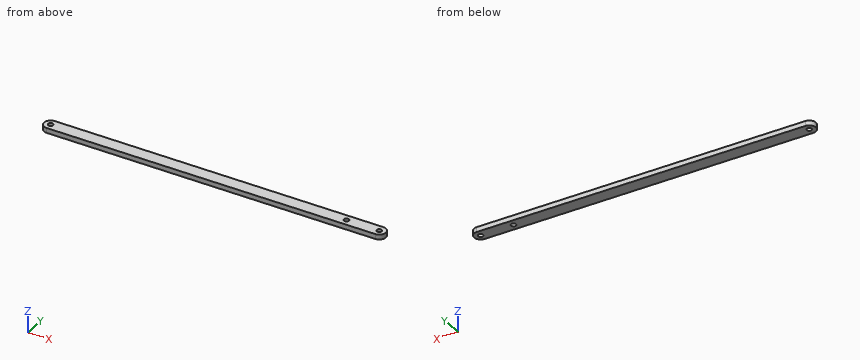
```python
from build123d import *

# Parameters (mm, degrees)
SKETCH1_R           = 3
BOSS_EXTRUDE1_DEPTH = 6
SCALE1_SCALE        = 0.5


with BuildPart() as part:
    # Sketch1 → Boss-Extrude1 (new body)
    with BuildSketch(Plane.XY):
        with BuildLine():
            Line((-200, 8), (200, 8))
            ThreePointArc((200, 8), (208, 0), (200, -8))
            Line((200, -8), (-200, -8))
            ThreePointArc((-200, -8), (-208, 0), (-200, 8))
        make_face()
        with Locations((-200, 0)):
            Circle(SKETCH1_R, mode=Mode.SUBTRACT)
        with Locations((200, 0)):
            Circle(SKETCH1_R, mode=Mode.SUBTRACT)
        with Locations((160, 0)):
            Circle(SKETCH1_R, mode=Mode.SUBTRACT)
    extrude(amount=-BOSS_EXTRUDE1_DEPTH)


with BuildPart() as part_1:
    # Scale1: scaled about (-0.694249163, 0, -3)
    add(part.part.scale(SCALE1_SCALE).moved(Location((-0.347124581, 0, -1.5))))


solid = part_1.part
```
CAD build for the part. Positions are in the model's coordinates, mm. Give positions to 0.01 mm unless a question says otherwise; leave off trailing zeros. Write each loop counter-clockwise with the first axis right and the second up, starting at its lowest first coordinate (ties: lowest second). Pieces come first, ordered by that corner, then holes. Notation, with made-up numbers: M 7.25,-38.5 L 32.25,-38.5 A15 ccw 32.25,-11.5 Z; hole C -19,50.25 d4. An arc over 180 degrees is marked long. Return JSON: item names as keys, results as strings. Group by question number.
(1) Drill centre lines: L1, parallel to X at y = 0.75, z = -4.35; L2, parallel to X at y = 3, z = -3.55; L3, parallel to X at y = -1.75, z = -2.65. Where is each one in solid material? Low to high. Write a range as [from, to].
(2) Band-saw the part on A-A (y = 0). Give the cut face in (x, z), and give its area (3 significant figures).
(3) Band-saw the part on B-B (z = -2.95). Give the cut face in (x, y), and give its area (3 significant figures).
Entries:
{
 "1": {"L1": "x = [-104.28, -101.65], [-99.05, 78.35], [80.95, 98.35], [100.95, 103.58]", "L2": "x = [-102.99, 102.3]", "L3": "x = [-103.94, 103.25]"},
 "2": {"outline": "M -104.35,-4.5 L -101.85,-4.5 L -101.85,-1.5 L -104.35,-1.5 Z; M -98.85,-4.5 L 78.15,-4.5 L 78.15,-1.5 L -98.85,-1.5 Z; M 81.15,-4.5 L 98.15,-4.5 L 98.15,-1.5 L 81.15,-1.5 Z; M 101.15,-4.5 L 103.65,-4.5 L 103.65,-1.5 L 101.15,-1.5 Z", "area": "597 mm^2"},
 "3": {"outline": "M -100.35,-4 L 99.65,-4 A4 ccw 99.65,4 L -100.35,4 A4 ccw Z; hole C -100.35,0 d3; hole C 79.65,0 d3; hole C 99.65,0 d3", "area": "1,630 mm^2"}
}
